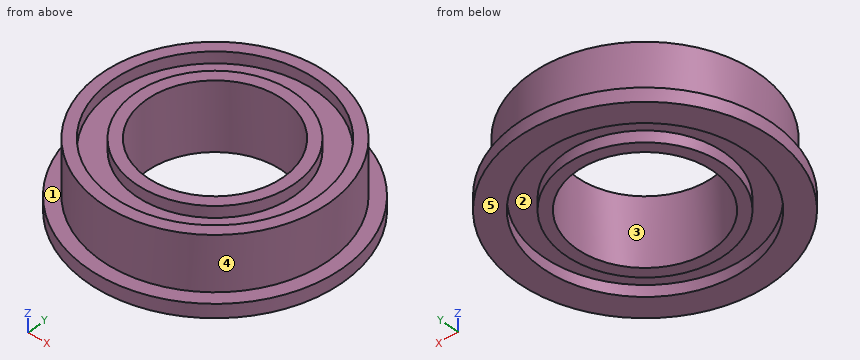
Autodesk Inventor part; units mm, degrees
ref_plane "YZ Plane" through (0, 0, 0) normal (1, 0, 0) x (0, 1, 0)
ref_plane "XZ Plane" through (0, 0, 0) normal (0, 1, 0) x (-1, 0, 0)
ref_plane "XY Plane" through (0, 0, 0) normal (0, 0, 1) x (1, 0, 0)
sketch "スケッチ1" plane through (0, 0, 0) normal (0, 0, 1) x (1, 0, 0)
  circle A0 centre (0, 0) radius 3
  circle A1 centre (0, 0) radius 5
  dimension "d0" = 6
  dimension "d1" = 10
extrude "押し出し1" add sketch "スケッチ1" along normal blind 3
sketch "スケッチ2" plane through (0, 0, 0) normal (0, 0, -1) x (-1, 0, 0)
  circle A0 centre (0, 0) radius 3
  circle A1 centre (0, 0) radius 5
  circle A2 centre (0, 0) radius 5.6
  dimension "d4" = 11.2
extrude "押し出し2" add sketch "スケッチ2" against normal blind 0.6 contours A2
sketch "スケッチ3" plane through (0, 0, 3) normal (0, 0, 1) x (1, 0, 0)
  circle A0 centre (0, 0) radius 3
  circle A1 centre (0, 0) radius 5
  circle A2 centre (0, 0) radius 4.5
  circle A3 centre (0, 0) radius 3.5
  dimension "d7" = 0.5
  dimension "d8" = 0.5
extrude "押し出し3" cut sketch "スケッチ3" against normal blind 0.5 contours A2
sketch "スケッチ4" plane through (0, 0, 0) normal (0, 0, -1) x (-1, 0, 0)
  circle A0 centre (0, 0) radius 3.5
  circle A1 centre (0, 0) radius 4.5
extrude "押し出し4" cut sketch "スケッチ4" against normal blind 0.5
sketch "スケッチ5" plane through (0, 0, 0) normal (0, 0, -1) x (-1, 0, 0)
  point P0 (0, 0)
properties part number "ベアリングHd6-D10-B3" material "鋼、炭素鋼"
The model under review builds one solid part; all positions refer to its coordinate system, in mm. Face numbers are marked on the shaded views. A direction names the side the tool comes from. Round coordinates to 2 decimals unless told otherwise and drop trailing zeros. Order: outer loops, then holes, each group sorted by start corner. A loop starts at its lowest first (then second) coordinate and runs counter-clockwise, first axis right, second up. Notation, with made-up numbers: (61.5, 55) -> (69.5, 55) arc R24 ccw to (69.5, 67) -> close; hole circle Ø1 at (5.25, 43.5). An arc over 180 degrees is marked (long way). One line per item, written item: value. Start each with the question number.
Q1. Take a section at A-A (x = 0). Write out the cut boundary in (y, z).
Q2. Clearance check with flat-ended pins moving along their axes: pin 1 Ø5.5 at (x, y) = (-0.5, -0.5) entering from +Z; pin 2 Ø1.5 at (y, z) = (-1.5, 1.5) entering from +X. State where each tip first meets the part, or that it passes through.
Q3. Take a section at C-C (z = 0.2). Write out the cut boundary in (x, y).
Q4. Wall thickness on line 1 (Y direction, x = 0, z = 0.2); line 2 (Y direction, x = 0, z = 2.2); line 3 (Y direction, x = -1.5, z = 0.2): over which ranges is each line inside the solid? List them lowest first.
Q5. Machinability: for the marked faces 1 and 2, which of the approach directions +Z, -Z, +X, -X, +Y, -Y give a long, thin tool a straight path to every point of the face, cutting with its end or side? Answer none if there is none.
Q6. Take a section at D-D (y = 4.75). Write out the cut boundary in (x, z), and give its area (3 significant figures).
Q7. Mouldability with a two-part tool opening along Y and no side actions: class the marked faces 3, 4 and 5 as released by +Y, released by -Y, zero draft, split by the parting line, or undercut.
Reported:
1. outline: (-5.6, 0) -> (-4.5, 0) -> (-4.5, 0.5) -> (-3.5, 0.5) -> (-3.5, 0) -> (-3, 0) -> (-3, 3) -> (-3.5, 3) -> (-3.5, 2.5) -> (-4.5, 2.5) -> (-4.5, 3) -> (-5, 3) -> (-5, 0.6) -> (-5.6, 0.6) -> close; (3, 0) -> (3.5, 0) -> (3.5, 0.5) -> (4.5, 0.5) -> (4.5, 0) -> (5.6, 0) -> (5.6, 0.6) -> (5, 0.6) -> (5, 3) -> (4.5, 3) -> (4.5, 2.5) -> (3.5, 2.5) -> (3.5, 3) -> (3, 3) -> close
2. pin 1: stops at z = 3
2. pin 2: stops at x = 4.94
3. outline: circle Ø11.2 at (0, 0); circle Ø7 at (0, 0); hole circle Ø9 at (0, 0); hole circle Ø6 at (0, 0)
4. line 1: y = -5.6 to -4.5, -3.5 to -3, 3 to 3.5, 4.5 to 5.6
4. line 2: y = -5 to -3, 3 to 5
4. line 3: y = -5.4 to -4.24, -3.16 to -2.6, 2.6 to 3.16, 4.24 to 5.4
5. face 1: +Z
5. face 2: -Z
6. outline: (-2.97, 0) -> (2.97, 0) -> (2.97, 0.6) -> (1.56, 0.6) -> (1.56, 3) -> (-1.56, 3) -> (-1.56, 0.6) -> (-2.97, 0.6) -> close
6. area: 11.1 mm2
7. face 3: undercut
7. face 4: split by the parting line
7. face 5: zero draft
